Read the model definition and answer for the solid it produces. Units are mm, in the model's axes. Round coordinates to 2 decimals unless told otherwise and drop trailing zeros. Order: outer loops, then holes, each group sorted by start corner. A loop starts at its lowest first (then second) coordinate and runs counter-clockwise, first axis right, second up. Notation, with made-up numbers: (-6, 69) -> (44, 69) arc R31 cw to (44, 107) -> close; hole circle Ø3 at (49, 42.5). An arc over 180 degrees is marked (long way). Answer as a JSON object with one key per item and string values. Group by question number.
Item 1: Section A-A, the plane z = 8 is taken. Write down the section's boundary in (x, y), plus the area to 3 significant figures.
Item 2: Section C-C, the plane x = -1 is taken. Write down the section's boundary in (y, z).
Item 3: Section B-B, the plane y = 10 is taken. Write down the section's boundary in (x, z), plus the area to 4 significant figures.
Item 4: Given P1, Ø2, axis at x = -2, y = 43, coming from the +Z side; P2, Ø1, axis at x = 4, z = 6, coming from the +Y side, each flat-ended and moving along its own axis, determine where each tip first touches the part or whether it passes through.
Item 5: Consider probe 1 along X at (y, z) = (190, 8); probe 2 along Z at (x, y) = (5.25, -140); probe 3 along X at (y, z) = (72, 11). Determine where each line is inside the solid, lowest interval first. Write a range as from..to.
from build123d import *

# Parameters (mm, degrees)
F1_DEPTH = 230


with BuildPart() as f1:
    # F0 (on Front) → F1 (new body, symmetric)
    with BuildSketch(Plane.XZ):
        Polygon((-9, 0), (0, 0), (9, 0), (9, 12.5), (4.5, 12.5), (4.5, 10.5), (6.25, 10.5), (6.25, 5), (4.75, 5), (4.75, 2.5), (0, 2.5), (-4.75, 2.5), (-4.75, 5), (-6.25, 5), (-6.25, 10.5), (-4.5, 10.5), (-4.5, 12.5), (-9, 12.5), align=None)
    extrude(amount=F1_DEPTH, both=True)


solid = f1.part
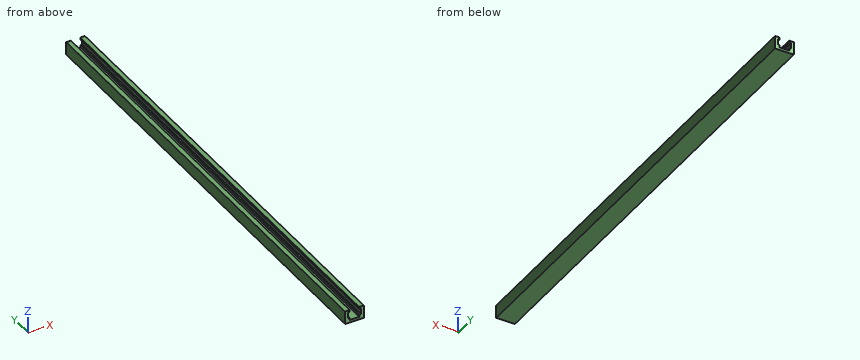
Values found:
{
 "1": {"outline": "(-9, -230) -> (-6.25, -230) -> (-6.25, 230) -> (-9, 230) -> close; (6.25, -230) -> (9, -230) -> (9, 230) -> (6.25, 230) -> close", "area": "2,530 mm2"},
 "2": {"outline": "(-230, 0) -> (230, 0) -> (230, 2.5) -> (-230, 2.5) -> close"},
 "3": {"outline": "(-9, 0) -> (9, 0) -> (9, 12.5) -> (4.5, 12.5) -> (4.5, 10.5) -> (6.25, 10.5) -> (6.25, 5) -> (4.75, 5) -> (4.75, 2.5) -> (-4.75, 2.5) -> (-4.75, 5) -> (-6.25, 5) -> (-6.25, 10.5) -> (-4.5, 10.5) -> (-4.5, 12.5) -> (-9, 12.5) -> close", "area": "114.5 mm2"},
 "4": {"P1": "z = 2.5", "P2": "through"},
 "5": {"probe 1": "-9..-6.25, 6.25..9", "probe 2": "0..5, 10.5..12.5", "probe 3": "-9..-4.5, 4.5..9"}
}
